Geometry check sheet. Reference: the model listing, model coordinates, mm. A direction names the side the tool comes from. Give positions to 0.01 mm unless a question says otherwise; leave off trailing zeros. Loops run counter-clockwise (first coordinate to the right, second up) from the corner with the lowest first, then second, coordinate; pieces in that order, holes last. Notation, with made-up numbers: (4, 22.5) - (18, 22.5) arc R17 ccw to (18, 42.5) - close; hole circle Ø9 at (-34.75, 65). An arc over 180 degrees is marked (long way). Use a Markdown table: item, result. Add a question column.
1. Cross-section at B-B on y = -11. Enter the section's corners in (x, z), and give its area (3 significant figures).
2. Depth check by flat-ended pin: P1, Ø5, axis at y = 0, z = 12.5, coming from the -X side; P2, Ø3, axis at x = 18.2, z = 10, coming from the +Y side; P3, Ø8, axis at x = -19, z = 6.5, coming from the +Y side; P4, Ø8, axis at x = 6.5, y = -7.5, coming from the +Z side. Enter the tip coordinate at first touch or a pass-through.
3. Cross-section at D-D on x = 0.5. Enter the section's corners in (y, z).
4. Draft check along Z on faces 6 (the flat face through (-4, -16, 0)), 7 (the flat face through (-4, -16, 20)), 8 (the cylindrical face through (-14.8, -12.8, 10.1)). Enter one of: pulls with the +Z half, pulls with the -Z half, needs draft (parallel to the pull), parting line crosses it, or undercut.
5. Cross-section at A-A on y = -6. Enter the section's corners in (x, z).
6. Set-up check for faces 1 (the flat face through (1, -17.5, 10)), 2 (the flat face through (-11.448, 0, 10)), 3 (the flat face through (21, -8.4, 10)), 4 (the flat face through (-21.448, -13, 10)), 5 (the cylindrical face through (20.2, -12.8, 10.1)): record each of +Z, -Z, +X, -X, +Y, -Y from which the full face is reachable in a straight line by a thin tool's end or side.
7. Material ranges on L1, parallel to Z at x = 18, y = -15.25; L2, parallel to X at y = -9, z = 19; L3, parallel to Y at x = 5, z = 5.25, recorded low to high.
8. Cross-section at C-C on z = 10. Enter the section's corners in (x, y), and give its area (3 significant figures).
from build123d import *

# Parameters (mm, degrees)
SKETCH1_W           = 25
SKETCH1_H           = 25.5
SKETCH1_R           = 11
SKETCH1_W_2         = 10
SKETCH1_H_2         = 9.1
BOSS_EXTRUDE1_DEPTH = 20
SKETCH2_R           = 2
CUT_EXTRUDE1_DEPTH  = 9


with BuildPart() as part:
    # Sketch1 → Boss-Extrude1 (new body)
    # profile 1 of 3: a face of its own
    with BuildSketch(Plane.XY):
        with Locations((1.051746227, -4.75)):
            Rectangle(SKETCH1_W, SKETCH1_H)
        with Locations((1.051746227, -6)):
            Circle(SKETCH1_R, mode=Mode.SUBTRACT)
    # profile 2 of 3: a face of its own
    with BuildSketch(Plane.XY):
        with Locations((-16.448253773, -12.95)):
            Rectangle(SKETCH1_W_2, SKETCH1_H_2)
    # profile 3 of 3: a face of its own
    with BuildSketch(Plane.XY):
        with Locations((18.551746227, -12.95)):
            Rectangle(SKETCH1_W_2, SKETCH1_H_2)
    extrude(amount=BOSS_EXTRUDE1_DEPTH)

    # Sketch2 → Cut-Extrude1 (cut)
    with BuildSketch(Plane(origin=(0, -8.4, 0), x_dir=(1, 0, 0), z_dir=(0, 1, 0))):
        with Locations(Location((-16.798835848, -10, 0), (0, 0, 180))):
            Circle(SKETCH2_R)
        with Locations(Location((18.201164152, -10, 0), (0, 0, 180))):
            Circle(SKETCH2_R)
    extrude(amount=-CUT_EXTRUDE1_DEPTH, mode=Mode.SUBTRACT)


solid = part.part
Values found:
| question | item | result |
|---|---|---|
| 1 | outline | (-21.45, 0) - (-8.75, 0) - (-8.75, 20) - (-21.45, 20) - close; (10.85, 0) - (23.55, 0) - (23.55, 20) - (10.85, 20) - close; hole circle Ø4 at (-16.8, 10); hole circle Ø4 at (18.2, 10) |
| 1 | area | 483 mm2 |
| 2 | P1 | stops at x = -11.45 |
| 2 | P2 | stops at y = -17.4 |
| 2 | P3 | stops at y = -8.4 |
| 2 | P4 | passes through |
| 3 | outline | (-17.5, 0) - (-16.99, 0) - (-16.99, 20) - (-17.5, 20) - close; (4.99, 0) - (8, 0) - (8, 20) - (4.99, 20) - close |
| 4 | face 6 | pulls with the -Z half |
| 4 | face 7 | pulls with the +Z half |
| 4 | face 8 | undercut |
| 5 | outline | (-11.45, 0) - (-9.95, 0) - (-9.95, 20) - (-11.45, 20) - close; (12.05, 0) - (13.55, 0) - (13.55, 20) - (12.05, 20) - close |
| 6 | face 1 | +Z, -Z, +X, -X, -Y |
| 6 | face 2 | +Z, -Z, -X, +Y |
| 6 | face 3 | +Z, -Z, +X, +Y |
| 6 | face 4 | +Z, -Z, -X, +Y, -Y |
| 6 | face 5 | +Y |
| 7 | L1 | z = 0 to 8.01, 11.99 to 20 |
| 7 | L2 | x = -21.45 to -9.53, 11.63 to 23.55 |
| 7 | L3 | y = -17.5 to -16.27, 4.27 to 8 |
| 8 | outline | (-21.45, -17.5) - (23.55, -17.5) - (23.55, -8.4) - (20.2, -8.4) - (20.2, -17.4) - (16.2, -17.4) - (16.2, -8.4) - (13.55, -8.4) - (13.55, 8) - (-11.45, 8) - (-11.45, -8.4) - (-14.8, -8.4) - (-14.8, -17.4) - (-18.8, -17.4) - (-18.8, -8.4) - (-21.45, -8.4) - close; hole circle Ø22 at (1.05, -6) |
| 8 | area | 367 mm2 |
